```python
from build123d import *

# Parameters (mm, degrees)
SKETCH_1_W          = 184
SKETCH_1_H          = 94
SKETCH_1_W_2        = 164
SKETCH_1_H_2        = 74
EXTRUDE_1_DEPTH     = 192
SKETCH_2_W          = 184
SKETCH_2_H          = 94
EXTRUDE_2_DEPTH     = 10
CUT_EXTRUDE_1_REACH = 234.732
CUT_EXTRUDE_2_REACH = 272.054
CUT_EXTRUDE_3_DEPTH = 10
CUT_EXTRUDE_4_DEPTH = 10
SKETCH_8_W          = 5
SKETCH_8_H          = 26.959910705
EXTRUDE_4_DEPTH     = 10
SKETCH_9_W          = 52
SKETCH_9_H          = 10
SKETCH_9_W_2        = 23
SKETCH_9_W_3        = 47
CUT_EXTRUDE_5_DEPTH = 10
FILLET_1_R          = 10


with BuildPart() as part:
    # 草图1 → 凸台-拉伸1 (new body)
    with BuildSketch(Plane.XY):
        Rectangle(SKETCH_1_W, SKETCH_1_H)
        Rectangle(SKETCH_1_W_2, SKETCH_1_H_2, mode=Mode.SUBTRACT)
    extrude(amount=-EXTRUDE_1_DEPTH)

    # 草图2 → 凸台-拉伸2 (add)
    with BuildSketch(Plane(origin=(0, 0, -192), x_dir=(-1, 0, 0), z_dir=(0, 0, -1))):
        Rectangle(SKETCH_2_W, SKETCH_2_H)
    extrude(amount=-EXTRUDE_2_DEPTH)

    # 草图3 → 切除-拉伸1 (cut, up to next)
    with BuildSketch(Plane(origin=(0, 47, 0), x_dir=(1, 0, 0), z_dir=(0, 1, 0)), mode=Mode.PRIVATE) as cut_extrude_1_sk1:
        with BuildLine():
            Line((35, 140), (35, 40))
            ThreePointArc((35, 40), (21.5, 26.5), (8, 40))
            Line((8, 40), (8, 140))
            ThreePointArc((8, 140), (21.5, 153.5), (35, 140))
        make_face()
    cut_extrude_1_tool1 = extrude(cut_extrude_1_sk1.sketch, amount=-CUT_EXTRUDE_1_REACH, mode=Mode.PRIVATE) & part.part
    # 草图3 → 切除-拉伸1 (cut, up to next)
    with BuildSketch(Plane(origin=(0, 47, 0), x_dir=(1, 0, 0), z_dir=(0, 1, 0)), mode=Mode.PRIVATE) as cut_extrude_1_sk2:
        with BuildLine():
            Line((-59, 42.5), (-59, 137.5))
            ThreePointArc((-59, 137.5), (-51.5, 145), (-44, 137.5))
            Line((-44, 137.5), (-44, 42.5))
            ThreePointArc((-44, 42.5), (-51.5, 35), (-59, 42.5))
        make_face()
    cut_extrude_1_tool2 = extrude(cut_extrude_1_sk2.sketch, amount=-CUT_EXTRUDE_1_REACH, mode=Mode.PRIVATE) & part.part
    add(cut_extrude_1_tool1.solids().sort_by_distance((21.5, 47, -90))[0], mode=Mode.SUBTRACT)
    add(cut_extrude_1_tool2.solids().sort_by_distance((-51.5, 47, -90))[0], mode=Mode.SUBTRACT)

    # 草图4 → 切除-拉伸2 (cut, up to next)
    with BuildSketch(Plane(origin=(92, 0, 0), x_dir=(0, 0, -1), z_dir=(1, 0, 0)), mode=Mode.PRIVATE) as cut_extrude_2_sk1:
        with BuildLine():
            Line((15, 9.5), (15, -9.5))
            ThreePointArc((15, -9.5), (16.171572875, -12.328427125), (19, -13.5))
            Line((19, -13.5), (161, -13.5))
            ThreePointArc((161, -13.5), (163.828427125, -12.328427125), (165, -9.5))
            Line((165, -9.5), (165, 9.5))
            ThreePointArc((165, 9.5), (163.828427125, 12.328427125), (161, 13.5))
            Line((161, 13.5), (19, 13.5))
            ThreePointArc((19, 13.5), (16.171572875, 12.328427125), (15, 9.5))
        make_face()
    cut_extrude_2_tool1 = extrude(cut_extrude_2_sk1.sketch, amount=-CUT_EXTRUDE_2_REACH, mode=Mode.PRIVATE) & part.part
    add(cut_extrude_2_tool1.solids().sort_by_distance((92, 0, -90))[0], mode=Mode.SUBTRACT)

    # 草图5 → 切除-拉伸3 (cut)
    with BuildSketch(Plane(origin=(0, 47, 0), x_dir=(1, 0, 0), z_dir=(0, 1, 0))):
        with BuildLine():
            ThreePointArc((35, 40), (21.5, 26.5), (8, 40))
            Line((8, 40), (8, 0))
            Line((8, 0), (35, 0))
            Line((35, 0), (35, 40))
        make_face()
        with BuildLine():
            Line((-59, 0), (-44, 0))
            Line((-44, 0), (-44, 42.5))
            ThreePointArc((-44, 42.5), (-51.5, 35), (-59, 42.5))
            Line((-59, 42.5), (-59, 0))
        make_face()
    extrude(amount=-CUT_EXTRUDE_3_DEPTH, mode=Mode.SUBTRACT)

    # 草图7 → 切除-拉伸4 (cut)
    with BuildSketch(Plane(origin=(92, 0, 0), x_dir=(0, 0, -1), z_dir=(1, 0, 0))):
        Polygon((18.435104252, 13.459910705), (-12.830882311, 13.459910705), (-16.882855926, -13.5), (19, -13.5), align=None)
    extrude(amount=-CUT_EXTRUDE_4_DEPTH, mode=Mode.SUBTRACT)

    # 草图8 → 凸台-拉伸4 (add)
    with BuildSketch(Plane(origin=(92, 0, 0), x_dir=(0, 0, -1), z_dir=(1, 0, 0))):
        with Locations((2.5, -0.020044647)):
            Rectangle(SKETCH_8_W, SKETCH_8_H)
    extrude(amount=-EXTRUDE_4_DEPTH)

    # 草图9 → 切除-拉伸5 (cut)
    with BuildSketch(Plane(origin=(0, 47, 0), x_dir=(1, 0, 0), z_dir=(0, 1, 0))):
        with Locations((-18, 5)):
            Rectangle(SKETCH_9_W, SKETCH_9_H)
        with Locations((-70.5, 5)):
            Rectangle(SKETCH_9_W_2, SKETCH_9_H)
        with Locations((58.5, 5)):
            Rectangle(SKETCH_9_W_3, SKETCH_9_H)
    extrude(amount=-CUT_EXTRUDE_5_DEPTH, mode=Mode.SUBTRACT)

    # 圆角1
    fillet_1_edges = [part.edges().sort_by_distance(p)[0] for p in [
        (-92, 47, -96),
        (92, 47, -96),
        (92, -47, -96),
    ]]
    fillet(fillet_1_edges, radius=FILLET_1_R)


solid = part.part
```
Read the model definition and answer for the solid it produces. Units are mm, in the model's axes. A direction names the side the tool comes from. Give positions to 0.01 mm unless a question says otherwise; leave off trailing zeros. Write each loop counter-clockwise with the first axis right and the second up, starting at its lowest first coordinate (ties: lowest second). Pieces come first, ordered by that corner, then holes. Notation, with made-up numbers: M 74.25,19.25 L 107.25,19.25 A14 ccw 107.25,45.25 Z; hole C -29.5,18 d11. An arc over 180 degrees is marked long. Put each result on its own line as item: value. Start each with the question number.
1. Consider line 1 along Y through (x, z) = (-79.5, -90); line 2 along X through (y, z) = (17, -56); line 3 along X through (y, z) = (39, -109.5). Determine where each line is inside the solid, lowest interval first.
2. Which of the six approach directions +Z, -Z, +X, -X, +Y, -Y give full straight-line access (tool end or side, diameter ignored) to faces 5 (the flat face through (87, 13.5, -91)), 6 (the flat face through (-59, 42, -75)), 7 (the flat face through (1, 1, -182)), 8 (the cylindrical face through (88.99, -44.15, -94.66)), 9 (the flat face through (-1, 1, -192))?
3. The part is cut by section B-B, the plane x = -51.5. Give the vertices of the cut face in (y, z).
4. The part is cut by section A-A, the plane z = -81.5. Give the vertices of the cut face in (x, y).
5. Each of these flat-tipped pins is pushed along its axis until it touches: pin 1 Ø5 at (x, z) = (88, -61.5) entering from +Y; pin 2 Ø3 at (x, y) = (59, 40) entering from +Z; pin 3 Ø11 at (x, z) = (89, -97) entering from -Y. Where does it stop, or does it pass through?
6. For a pull along Y with two mould halves and no side action, classify faces 1 (the flat face through (-1, 37, -95)), 2 (the cylindrical face through (88.99, 44.15, -97.34)), 3 (the cylindrical face through (21.203, 42.07, -153.497)), 4 (the flat face through (87, 0, -165)) as released by +Y, released by -Y, zero draft, split by the parting line, or undercut.
7. The part is cut by section C-C, the plane x = 21.5. Give the vertices of the cut face in (y, z), and give its area (4 significant figures).
Final values:
1. line 1: y = -47 to -37, 37 to 47
1. line 2: x = -92 to -82, 82 to 92
1. line 3: x = -91.8 to -59, -44 to 8, 35 to 91.8
2. face 5: +X
2. face 6: +Z, +Y
2. face 7: +Z
2. face 8: +Z, -Z, +X, -Y
2. face 9: -Z, +X, -X, +Y, -Y
3. outline: M -47,-192 L 47,-192 L 47,-145 L 37,-145 L 37,-182 L -37,-182 L -37,0 L -47,0 Z
4. outline: M -92,-47 L 82,-47 A10 ccw 92,-37 L 92,-13.5 L 82,-13.5 L 82,-37 L -82,-37 L -82,37 L -59,37 L -59,47 L -82,47 A10 ccw -92,37 Z; M -44,37 L 8,37 L 8,47 L -44,47 Z; M 35,37 L 82,37 L 82,13.5 L 92,13.5 L 92,37 A10 ccw 82,47 L 35,47 Z
5. pin 1: stops at y = 46.37
5. pin 2: stops at z = -10
5. pin 3: stops at y = -46.89
6. face 1: undercut
6. face 2: released by +Y
6. face 3: zero draft
6. face 4: undercut
7. outline: M -47,-192 L 47,-192 L 47,-153.5 L 37,-153.5 L 37,-182 L -37,-182 L -37,0 L -47,0 Z
7. area: 3,045 mm²
